For this review, use the dimensioned drawing (mm, ordinates from the lowest corner) and the shaded views. Round coordinates to 2 decimals unless told otherwise and drop trailing zeros. Loops run counter-clockwise (first coordinate to the right, second up) from the corner with the lowest first, then second, coordinate; pieces in that order, holes last. Notation, with made-up numbers: M 33,34 L 55,34 A17 cw 55,40 Z; hole C -39.75,58.5 d2. An arc over 180 degrees is marked long. Answer as a JSON object with one key per item and string values. Group by question number.
Item 1: Insertion check: P1, Ø10, axis at x = 20.35, y = 20.35, coming from the -Z side; P2, Ø1, axis at x = 20, z = 1.5, coming from the +Y side. Each pin has a flat end and moves straight along its axis. Give the tip position at first contact, or say it passes through.
Item 2: Consider section A-A (x = 20.35). Give the boundary of the cut face in (y, z), and give its area (4 significant figures).
Item 3: Consider section C-C (z = 2.05). Give the boundary of the cut face in (x, y), and give its area (3 significant figures).
Item 4: The part is to be moulded in two halves that separate along X. For the marked faces 1, 2 and 3, say which applies: +X half, -X half, draft (parallel to the pull), parting line (faces both ways), or undercut.
Item 5: Consider section D-D (x = 5.35). Give the boundary of the cut face in (y, z), and give its area (3 significant figures).
Item 6: To check wall thickness, follow line 1 (Y direction, x = 20.35, z = 0.25); line 2 (Y direction, x = 20.35, z = 0.8); line 3 (X direction, y = 21, z = 0.7). State the ranges of each line that lie inside material, in increasing order.
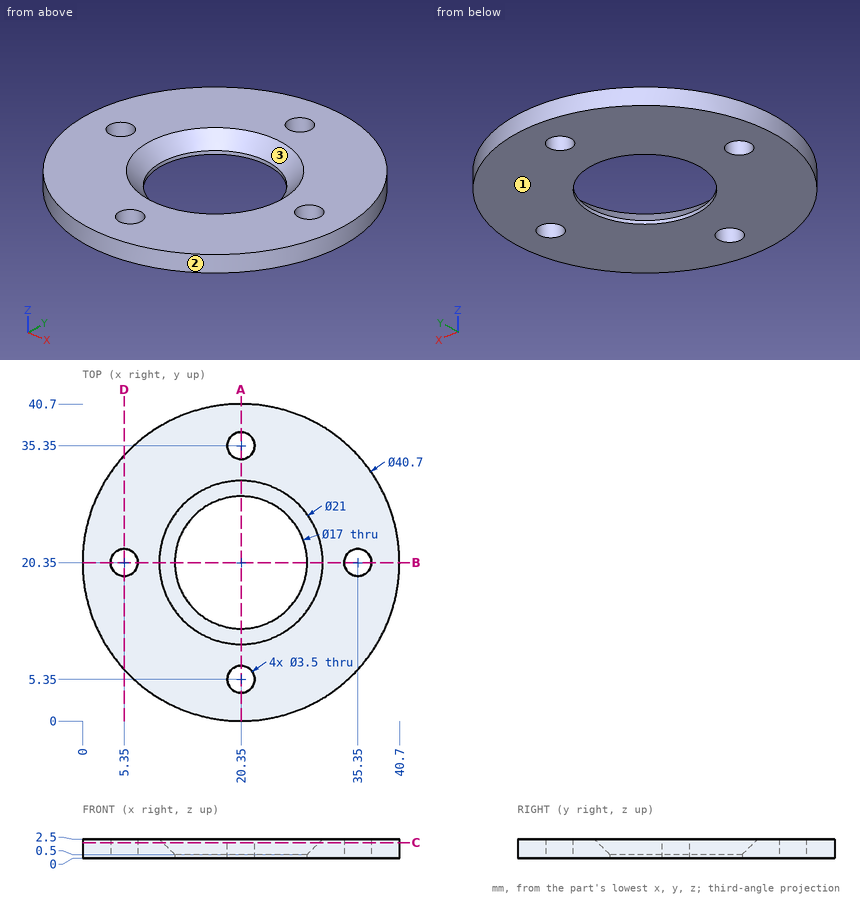
Geometry results:
{
 "1": {"P1": "passes through", "P2": "stops at y = 40.7"},
 "2": {"outline": "M 0,0 L 3.6,0 L 3.6,2.5 L 0,2.5 Z; M 7.1,0 L 11.85,0 L 11.85,0.5 L 9.85,2.5 L 7.1,2.5 Z; M 28.85,0 L 33.6,0 L 33.6,2.5 L 30.85,2.5 L 28.85,0.5 Z; M 37.1,0 L 40.7,0 L 40.7,2.5 L 37.1,2.5 Z", "area": "37.75 mm^2"},
 "3": {"outline": "C 20.35,20.35 d40.7; hole C 5.35,20.35 d3.5; hole C 20.35,20.35 d20.1; hole C 20.35,5.35 d3.5; hole C 20.35,35.35 d3.5; hole C 35.35,20.35 d3.5", "area": "945 mm^2"},
 "4": {"face 1": "draft", "face 2": "parting line", "face 3": "undercut"},
 "5": {"outline": "M 6.6,0 L 18.6,0 L 18.6,2.5 L 6.6,2.5 Z; M 22.1,0 L 34.1,0 L 34.1,2.5 L 22.1,2.5 Z", "area": "60.0 mm^2"},
 "6": {"line 1": "y = 0 to 3.6, 7.1 to 11.85, 28.85 to 33.6, 37.1 to 40.7", "line 2": "y = 0 to 3.6, 7.1 to 11.55, 29.15 to 33.6, 37.1 to 40.7", "line 3": "x = 0.01 to 3.73, 6.97 to 11.67, 29.03 to 33.73, 36.97 to 40.69"}
}
